Source: three-view drawing plus pictorial views. Frame: mm from the lowest corner of the part. A direction names the side the tool comes from. Round coordinates to 2 decimals unless told otherwise and drop trailing zeros. Write each loop counter-clockwise with the first axis right and the second up, starting at its lowest first coordinate (ties: lowest second). Pieces come first, ordered by that corner, then holes. Notation, with made-up numbers: M -38.5,-32 L -9.5,-32 A27 ccw -9.5,2 Z; hole C -3,56 d6. An arc over 180 degrees is marked long. Answer as CSV lines item,"result". Start each with the question number.
Q1. Section query D-D on y = 4.75. Output: boundary loops of the cut face in (x, z).
Q2. First-contact query: pin 1 (6 mm diameter, centred on x = 16.5, z = 3, fed in from +Y) (1 decimal); pin 2 (0.5 mm diameter, centred on x = 0.5, z = 12.5, fed in from +Y); pin 3 (5 mm diameter, centred on x = 17.5, y = 3.5, fed in from -Z); pin 4 (2 mm diameter, centred on x = 11.5, y = 7.5, fed in from -Z). Flat tips, straight axial feed; report the tip coordinate or a pass-through.
Q3. Section query B-B on z = 22.5. Output: boundary loops of the cut face in (x, y) (1 decimal).
Q4. Section query A-A on y = 7.25. Output: boundary loops of the cut face in (x, z).
Q5. Mould query, pull axis Z, two halves, no side actions, for the marked faces 3, 4, 5 and 6. Classes: pulls with the +Z half, pulls with the -Z half, needs draft (parallel to the pull), parting line crosses it, or undercut.
Q6. Ray query, probe 1 along X at (y, z) = (6, 10.5); probe 2 along Y at (x, z) = (16.5, 22.5) (1 decimal). Return the intervals inside material, ascending.
Q7. Reachability of the marked faces 1 and 2 from +Z, -Z, +X, -X, +Y, -Y: full face, straight path, thin tool, end or side. Return the list, or none.
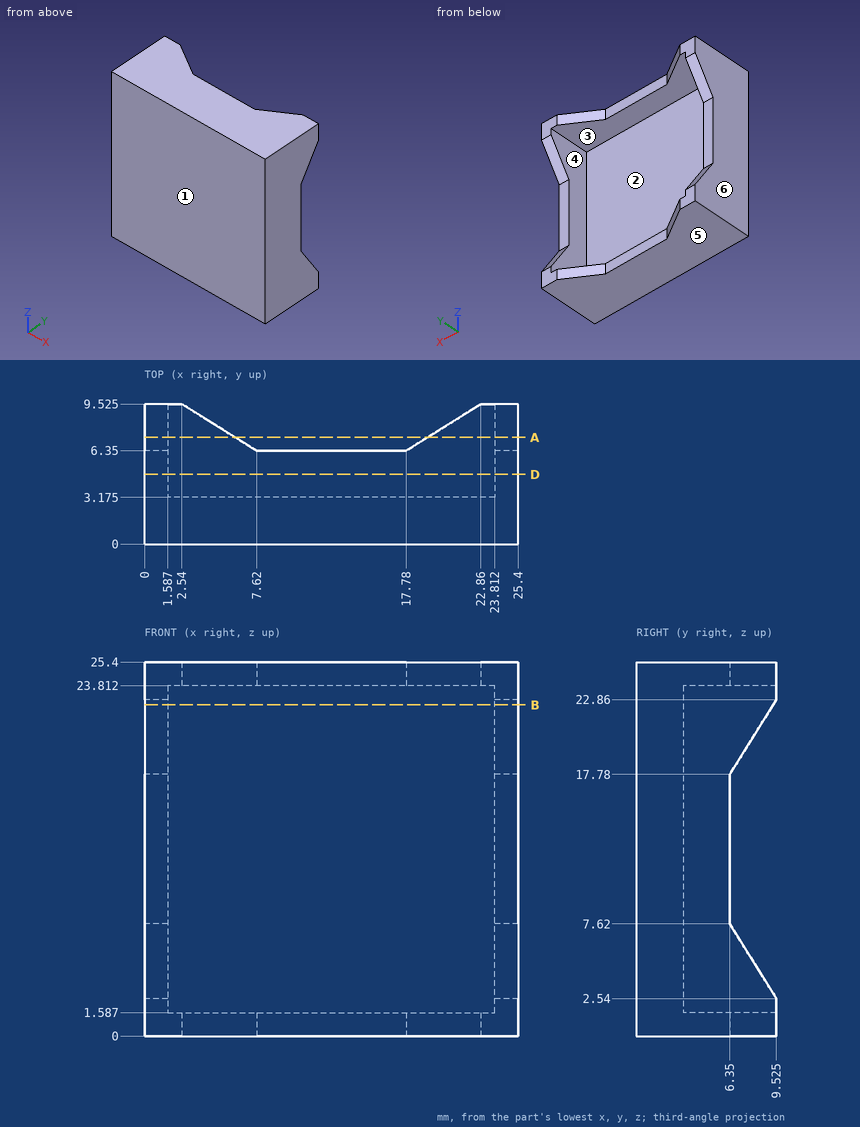
Entries:
1,outline,"M 0,0 L 25.4,0 L 25.4,25.4 L 0,25.4 Z; hole M 1.59,1.59 L 23.81,1.59 L 23.81,23.81 L 1.59,23.81 Z"
2,pin 1,"stops at y = 7.2"
2,pin 2,"stops at y = 6.35"
2,pin 3,"stops at z = 0"
2,pin 4,"passes through"
3,outline,"M 0,0 L 25.4,0 L 25.4,9.3 L 23.8,9.3 L 23.8,3.2 L 1.6,3.2 L 1.6,9.3 L 0,9.3 Z"
4,outline,"M 0,0 L 6.18,0 L 6.18,1.59 L 1.59,1.59 L 1.59,6.18 L 0,6.18 Z; M 0,19.22 L 1.59,19.22 L 1.59,23.81 L 6.18,23.81 L 6.18,25.4 L 0,25.4 Z; M 19.22,0 L 25.4,0 L 25.4,6.18 L 23.81,6.18 L 23.81,1.59 L 19.22,1.59 Z; M 19.22,23.81 L 23.81,23.81 L 23.81,19.22 L 25.4,19.22 L 25.4,25.4 L 19.22,25.4 Z"
5,face 3,"undercut"
5,face 4,"undercut"
5,face 5,"pulls with the -Z half"
5,face 6,"needs draft"
6,probe 1,"x = 0 to 1.59, 23.81 to 25.4"
6,probe 2,"y = 0 to 3.2"
7,face 1,"+Z, -Z, +X, -X, -Y"
7,face 2,"+Y"
